Answer from the drawing. Dimensions are ordinates in mm from the lowest x, y and z of the part. A direction names the side the tool comes from. Round coordinates to 2 decimals unless told otherwise and drop trailing zeros. Loops run counter-clockwise (first coordinate to the right, second up) from the corner with the lowest first, then second, coordinate; pieces in that order, holes last. Notation, with made-up numbers: (26, 22.5) - (57, 22.5) arc R28 ccw to (57, 51.5) - close; hole circle Ø11 at (2, 26.5). An arc over 180 degrees is marked (long way). Answer as CSV lines item,"result". Start each with the question number.
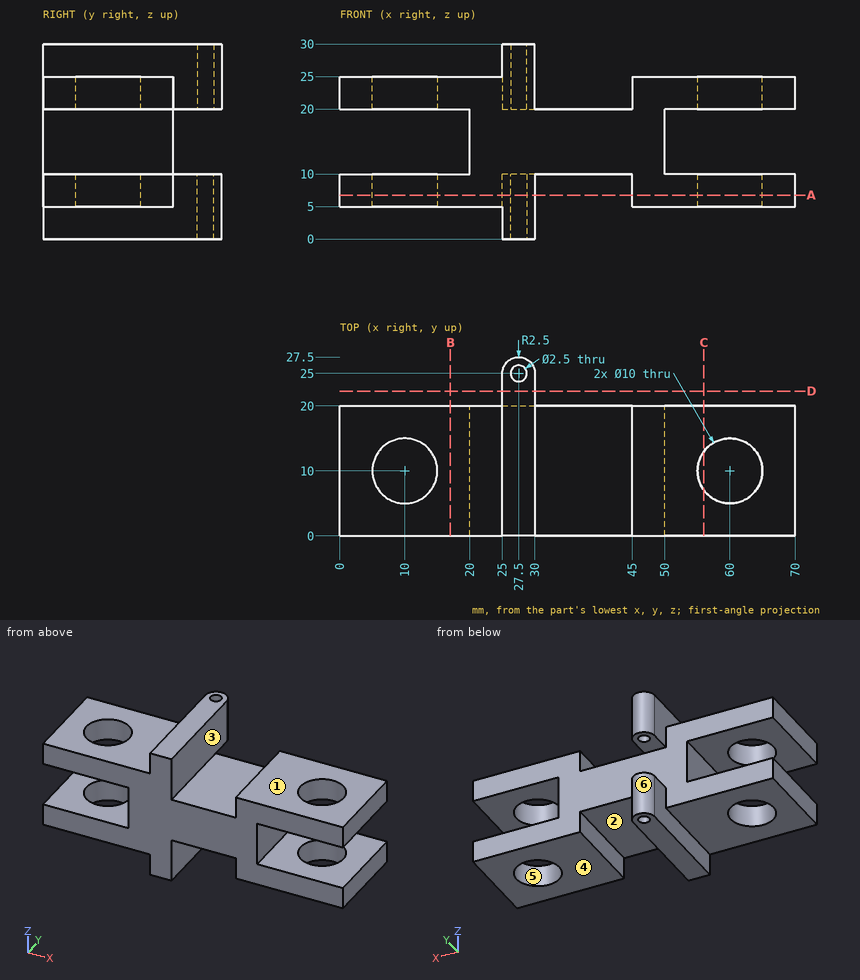
Item 1: Determine the mould class of the marked faces 4, 5 and 6 for opening direction Y: pulls with the +Y half, pulls with the -Y half, needs draft (parallel to the pull), parting line crosses it, or undercut.
Item 2: Flat-ended cylindrical pins translate along their axes: pin 1 Ø2 at (y, z) = (3, 26.5) entering from -X; pin 2 Ø8 at (x, y) = (10, 10) entering from -Z; pin 3 Ø6 at (x, y) = (34.5, 5) entering from -Z; pin 4 Ø6 at (x, y) = (59.5, 6.5) entering from +Z. Find the tip coordinate at first contact, or state that the pin passes through.
Item 3: Section D-D, the plane y = 22.25 is taken. Give the vertices of the cut face in (x, z), and give its area (3 significant figures).
Item 4: Section C-C, the plane x = 56 is taken. Give the vertices of the cut face in (y, z).
Item 5: Section A-A, the plane z = 6.75 is taken. Give the vertices of the cut face in (x, y).
Item 6: Which of the six approach directions +Z, -Z, +X, -X, +Y, -Y give full straight-line access (tool end or side, diameter ignored) to the marked faces 1, 2 and 3?
Item 7: Section B-B, the plane x = 17 is taken. Give the vertices of the cut face in (y, z), and give its area (3 significant figures).
Item 8: Find the intervals of material crossed by L1, parallel to Y at x = 27.5, z = 6.75; L2, parallel to Z at x = 25.5, y = 25.5; L3, parallel to Z at x = 61, y = 16.25, in increasing order.
Answer:
1,face 4,"needs draft"
1,face 5,"undercut"
1,face 6,"pulls with the +Y half"
2,pin 1,"stops at x = 25"
2,pin 2,"passes through"
2,pin 3,"stops at z = 10"
2,pin 4,"stops at z = 25"
3,outline,"(25, 0) - (30, 0) - (30, 10) - (25, 10) - close; (25, 20) - (30, 20) - (30, 30) - (25, 30) - close"
3,area,"100 mm²"
4,outline,"(0, 5) - (7, 5) - (7, 10) - (0, 10) - close; (0, 20) - (7, 20) - (7, 25) - (0, 25) - close; (13, 5) - (20, 5) - (20, 10) - (13, 10) - close; (13, 20) - (20, 20) - (20, 25) - (13, 25) - close"
5,outline,"(0, 0) - (30, 0) - (30, 25) arc R2.5 ccw to (25, 25) - (25, 20) - (0, 20) - close; (45, 0) - (70, 0) - (70, 20) - (45, 20) - close; hole circle Ø10 at (10, 10); hole circle Ø2.5 at (27.5, 25); hole circle Ø10 at (60, 10)"
6,face 1,"+Z, +X, +Y, -Y"
6,face 2,"-Z, +Y, -Y"
6,face 3,"+Z, +Y, -Y"
7,outline,"(0, 5) - (20, 5) - (20, 10) - (0, 10) - close; (0, 20) - (20, 20) - (20, 25) - (0, 25) - close"
7,area,"200 mm²"
8,L1,"y = 0 to 23.75, 26.25 to 27.5"
8,L2,"z = 0 to 10, 20 to 30"
8,L3,"z = 5 to 10, 20 to 25"
